For this review, use the dimensioned drawing (mm, ordinates from the lowest corner) and the shaded views. A direction names the side the tool comes from. Round coordinates to 2 decimals unless told otherwise and drop trailing zeros. Loops run counter-clockwise (first coordinate to the right, second up) from the corner with the lowest first, then second, coordinate; pieces in that order, holes last. Notation, with made-up numbers: M 13.25,81.25 L 23.25,81.25 A24 cw 23.25,106.25 Z; hole C 50.5,13 d3. An arc over 180 degrees is marked long. One line per item, written item: value. Start each with the question number.
Item 1: We need section A-A (x = 25.08). Write out the cut boundary in (y, z).
Item 2: Mouldability with a two-part tool opening along Z and no side actions: class the marked faces 1, 2 and 3 as released by +Z, released by -Z, zero draft, split by the parting line, or undercut.
Item 3: We need section C-C (y = 32.5). Write out the cut boundary in (x, z), then the cut area to 3 significant figures.
Item 4: We need section D-D (x = 72). Write out the cut boundary in (y, z).
Item 5: We need section B-B (y = 16.92). Write out the cut boundary in (x, z).
Item 6: For the marked faces 4 and 5, list the 3-axis set-ups (+Z, -Z, +X, -X, +Y, -Y) from which the entire face can be reached by the end or side of a thin tool; tool diameter is ignored.
Item 7: Clearance check with flat-ended pins moving along their axes: pin 1 (8 mm diameter, centred on x = 25.08, y = 16.92, fed in from +Z); pin 2 (5 mm diameter, centred on x = 66, z = 34, fed in from -Y). State where each tip first meets the part, or that it passes through.
Item 8: For line 1 along Z through (x, y) = (29, 33.5); line 2 along Y through (x, z) = (25, 74); line 3 along X through (y, z) = (16, 74), list the stretches that pass through material, from the lowest coordinate up.
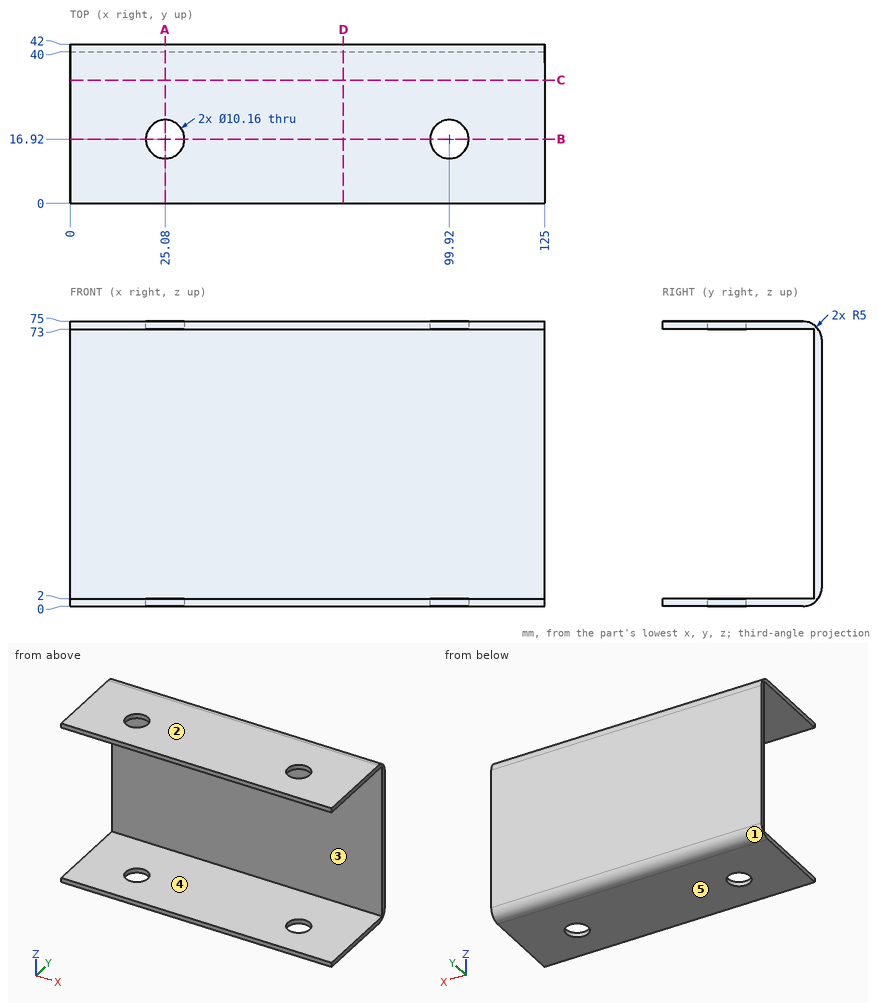
A:
1. outline: M 0,0 L 11.84,0 L 11.84,2 L 0,2 Z; M 0,73 L 11.84,73 L 11.84,75 L 0,75 Z; M 22,0 L 37,0 A5 ccw 42,5 L 42,70 A5 ccw 37,75 L 22,75 L 22,73 L 40,73 L 40,2 L 22,2 Z
2. face 1: released by -Z
2. face 2: released by +Z
2. face 3: undercut
3. outline: M 0,0 L 125,0 L 125,2 L 0,2 Z; M 0,73 L 125,73 L 125,75 L 0,75 Z
3. area: 500 mm2
4. outline: M 0,0 L 37,0 A5 ccw 42,5 L 42,70 A5 ccw 37,75 L 0,75 L 0,73 L 40,73 L 40,2 L 0,2 Z
5. outline: M 0,0 L 20,0 L 20,2 L 0,2 Z; M 0,73 L 20,73 L 20,75 L 0,75 Z; M 30.16,0 L 94.84,0 L 94.84,2 L 30.16,2 Z; M 30.16,73 L 94.84,73 L 94.84,75 L 30.16,75 Z; M 105,0 L 125,0 L 125,2 L 105,2 Z; M 105,73 L 125,73 L 125,75 L 105,75 Z
6. face 4: +X, -X, -Y
6. face 5: -Z, +X, -X, +Y, -Y
7. pin 1: through
7. pin 2: y = 40
8. line 1: 0 to 2, 73 to 75
8. line 2: 0 to 11.84, 22 to 40
8. line 3: 0 to 20.08, 30.08 to 94.92, 104.92 to 125
